from build123d import *

# Parameters (mm, degrees)
SKETCH1_W                         = 175
SKETCH1_H                         = 120
BOSS_EXTRUDE1_DEPTH               = 3.125
F_1_2_20_TAPPED_HOLE1_D           = 11.50874
F_1_2_20_TAPPED_HOLE1_DEPTH       = 30
F_1_2_20_TAPPED_HOLE1_CSINK_D     = 13.97
F_1_2_20_TAPPED_HOLE1_CSINK_ANGLE = 90
F_1_2_20_TAPPED_HOLE1_TIP         = 3.45757432


with BuildPart() as part:
    # Sketch1 → Boss-Extrude1 (new body)
    with BuildSketch(Plane(origin=(0, 0, 0), x_dir=(1, 0, 0), z_dir=(0, 1, 0))):
        with Locations((87.5, 60)):
            Rectangle(SKETCH1_W, SKETCH1_H)
    extrude(amount=BOSS_EXTRUDE1_DEPTH)

    # 1/2-20 Tapped Hole1
    with Locations(Plane(origin=(0, 3.125, 0), x_dir=(1, 0, 0), z_dir=(0, 1, 0))):
        with Locations((148.5, 93.5)):
            CounterSinkHole(F_1_2_20_TAPPED_HOLE1_D / 2, F_1_2_20_TAPPED_HOLE1_CSINK_D / 2, depth=F_1_2_20_TAPPED_HOLE1_DEPTH, counter_sink_angle=F_1_2_20_TAPPED_HOLE1_CSINK_ANGLE)
            with Locations((0, 0, -(F_1_2_20_TAPPED_HOLE1_DEPTH + F_1_2_20_TAPPED_HOLE1_TIP / 2))):  # 118° drill point
                Cone(0, F_1_2_20_TAPPED_HOLE1_D / 2, F_1_2_20_TAPPED_HOLE1_TIP, mode=Mode.SUBTRACT)


solid = part.part
Model file for the job. Use its own axes, mm. Coordinates: 2 decimals unless noted, no trailing zeros. Order: outer loops, then holes, each group sorted by start corner. A loop starts at its lowest first (then second) coordinate and runs counter-clockwise, first axis right, second up. Notation, with made-up numbers: M -5,12 L 52,12 A17 cw 52,40 Z; hole C 14,15.25 d9. An arc over 180 degrees is marked long. Return JSON: item names as keys, results as strings.
1. Saw through at A-A (z = -93.5). Give the cut face in (x, y) (3 decimals).
Ans:
{"outline": "M 0,0 L 142.746,0 L 142.746,1.894 L 141.515,3.125 L 0,3.125 Z; M 154.254,0 L 175,0 L 175,3.125 L 155.485,3.125 L 154.254,1.894 Z"}
2. Pull direction X, two halves, no side cores. Call faces 1 (the face through (143.184, 0.934, -91.296)), 2 (the face through (86, 3.125, -61)): +X half, -X half, draft (parallel to the pull), parting line (faces both ways), or undercut.
Ans:
{"face 1": "undercut", "face 2": "draft"}
3. Drill centre lines: probe 1 along Z at (x, y) = (148.5, 0.85); probe 2 along X at (y, z) = (0.6, -93.5). Where is each one in solid material? Low to high.
Ans:
{"probe 1": "-120 to -99.25, -87.75 to 0", "probe 2": "0 to 142.75, 154.25 to 175"}
4. Flat gauge pin, fed straight in: pin 1 (2 mm diameter, centred on x = 107.5, z = -40, fed in from -Y). Where does the tip first touch, or does it go through?
Ans:
{"pin 1": "y = 0"}
5. Saw through at B-B (x = 148.5). Give the cut face in (y, z) (3 decimals).
Ans:
{"outline": "M 0,-120 L 3.125,-120 L 3.125,-100.485 L 1.894,-99.254 L 0,-99.254 Z; M 0,-87.746 L 1.894,-87.746 L 3.125,-86.515 L 3.125,0 L 0,0 Z"}
